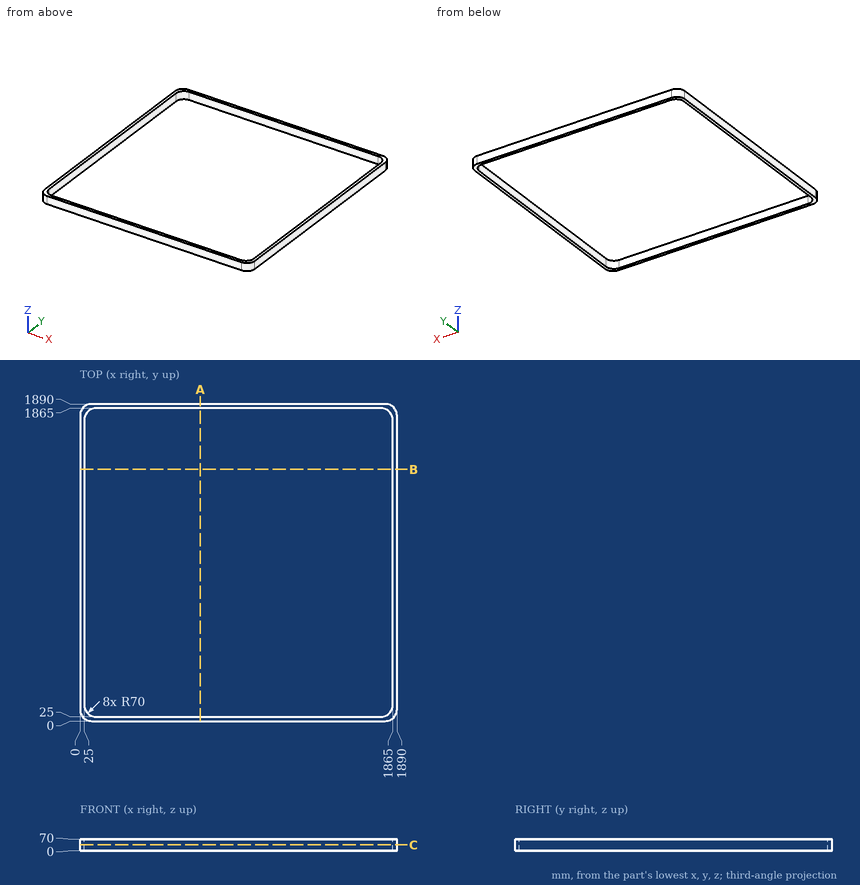
Can you work these out from the drawing? Everything is in mm from the part's minimum corner. Coordinates: 2 decimals unless noted, no trailing zeros. Write each loop counter-clockwise with the first axis right and the second up, starting at its lowest first coordinate (ties: lowest second). Pieces come first, ordered by that corner, then holes. Notation, with made-up numbers: (37.5, 53) -> (76.5, 53) arc R17 cw to (76.5, 74) -> close; hole circle Ø6 at (-4.5, 31.25). An arc over 180 degrees is marked (long way). Return JSON: item names as keys, results as strings.
(1) Imagine slicing it at C-C, the plane z = 35.5. Please give me the cut outline in (x, y), then the cut area to 4 significant figures.
Numbers:
{"outline": "(0, 70) arc R70 ccw to (70, 0) -> (1820, 0) arc R70 ccw to (1890, 70) -> (1890, 1820) arc R70 ccw to (1820, 1890) -> (70, 1890) arc R70 ccw to (0, 1820) -> close; hole (25, 95) arc R70 ccw to (95, 25) -> (1795, 25) arc R70 ccw to (1865, 95) -> (1865, 1795) arc R70 ccw to (1795, 1865) -> (95, 1865) arc R70 ccw to (25, 1795) -> close", "area": "186,500 mm2"}
(2) Imagine slicing it at A-A, the plane x = 718. Please give me the cut outline in (y, z).
Numbers:
{"outline": "(0, 0) -> (25, 0) -> (25, 70) -> (0, 70) -> close; (1865, 0) -> (1890, 0) -> (1890, 70) -> (1865, 70) -> close"}
(3) I need wall thicknesses on L1, parallel to X at y = 1118, z = 29; L2, parallel to Y at x = 1803, z = 40. Which ranges of each line are inside material? Lowest first, please.
Numbers:
{"L1": "x = 0 to 25, 1865 to 1890", "L2": "y = 0 to 25.46, 1864.54 to 1890"}
